Source: three-view drawing plus pictorial views. Frame: mm from the lowest corner of the part. A direction names the side the tool comes from. Coordinates: 2 decimals unless noted, no trailing zeros. Write each loop counter-clockwise with the first axis right and the second up, starting at its lowest first coordinate (ties: lowest second). Pieces come first, ordered by that corner, then holes. Notation, with made-up numbers: (-13, 81) - (42, 81) arc R16 ccw to (42, 103) - close; hole circle Ø4 at (-39.5, 26). An arc over 180 degrees is marked (long way). One line per item, written item: value.
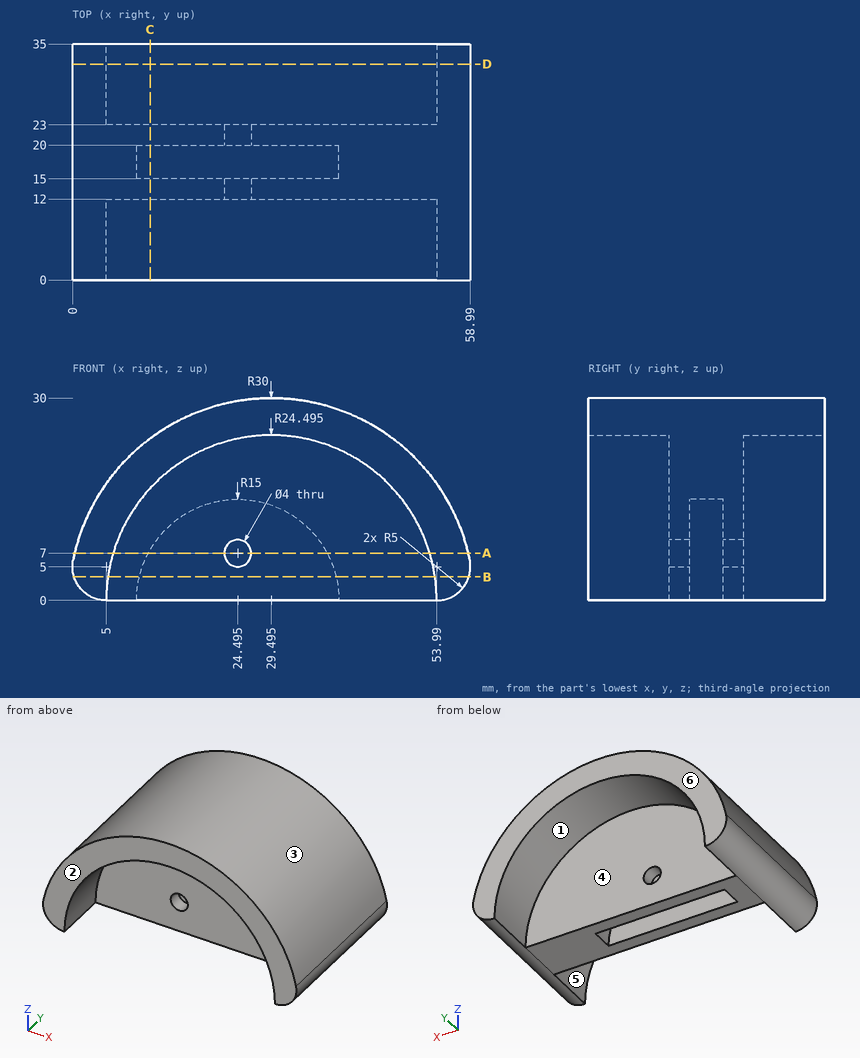
1) Reachability of the marked faces 4, 5 and 6 from +Z, -Z, +X, -X, +Y, -Y: full face, straight path, thin tool, end or side. Return the list, or none.
Values found:
face 4: -Z, +Y
face 5: -Z, -Y
face 6: +Z, -Z, +X, -X, +Y
2) Section query D-D on y = 32. Output: boundary loops of the cut face in (x, z) (1 decimal), then the cut area to 3 significant figures.
Values found:
outline: (0.1, 6) arc R5 ccw to (5, 0) arc R24.5 cw to (54, 0) arc R5 ccw to (58.9, 6) arc R30 ccw to start
area: 457 mm2
3) Material intervals for line 1 (Y direction, x = 30.5, z = 2); line 2 (Y direction, x = 50, z = 13.25); line 3 (X direction, y = 26, z = 17.75) (1 decimal), sorted ascending.
Values found:
line 1: 12 to 15, 20 to 23
line 2: 12 to 23
line 3: 5.3 to 12.6, 46.4 to 53.7
4) Section query A-A on z = 7. Output: boundary loops of the cut face in (x, y) (1 decimal).
Values found:
outline: (0.3, 0) - (6, 0) - (6, 12) - (22.5, 12) - (22.5, 15) - (11.2, 15) - (11.2, 20) - (22.5, 20) - (22.5, 23) - (6, 23) - (6, 35) - (0.3, 35) - close; (26.5, 12) - (53, 12) - (53, 0) - (58.7, 0) - (58.7, 35) - (53, 35) - (53, 23) - (26.5, 23) - (26.5, 20) - (37.8, 20) - (37.8, 15) - (26.5, 15) - close
5) Section query B-B on z = 3.5. Output: boundary loops of the cut face in (x, y).
Values found:
outline: (0.23, 0) - (5.25, 0) - (5.25, 12) - (53.74, 12) - (53.74, 0) - (58.76, 0) - (58.76, 35) - (53.74, 35) - (53.74, 23) - (5.25, 23) - (5.25, 35) - (0.23, 35) - close; hole (9.91, 15) - (39.08, 15) - (39.08, 20) - (9.91, 20) - close
6) Section query C-C on x = 11.5. Output: boundary loops of the cut face in (y, z), then the cut area to 3 significant figures.
Values found:
outline: (0, 16.62) - (12, 16.62) - (12, 0) - (15, 0) - (15, 7.49) - (20, 7.49) - (20, 0) - (23, 0) - (23, 16.62) - (35, 16.62) - (35, 24) - (0, 24) - close
area: 404 mm2
7) Draft query along X for the marked faces 1, 2 and 3. Return one class per face: released by +X, released by -X, zero draft, split by the parting line, or undercut.
Values found:
face 1: undercut
face 2: zero draft
face 3: split by the parting line
8) Contact query for flat-ended pins moving along their axis: P1, Ø3, axis at x = 48.5, z = 10, coming from the -Y side; P2, Ø4.5, axis at x = 23, z = 5, coming from the +Y side. Output: stop coordinate, or through.
Values found:
P1: y = 12
P2: y = 23
